from build123d import *

# Parameters (mm, degrees)
SKETCH1_W           = 94
SKETCH1_H           = 57
BOSS_EXTRUDE1_DEPTH = 1
BOSS_EXTRUDE3_DEPTH = 30
SKETCH5_W           = 0.7
SKETCH5_H           = 1
BOSS_EXTRUDE4_DEPTH = 92
SKETCH6_W           = 47
SKETCH6_H           = 10
CUT_EXTRUDE2_DEPTH  = 30
SKETCH7_W           = 10
SKETCH7_H           = 2
BOSS_EXTRUDE5_DEPTH = 2


with BuildPart() as part:
    # Sketch1 → Boss-Extrude1 (new body)
    with BuildSketch(Plane(origin=(0, 0, 0), x_dir=(1, 0, 0), z_dir=(0, 1, 0))):
        with Locations((-9.450515464, -3.911340206)):
            Rectangle(SKETCH1_W, SKETCH1_H)
    extrude(amount=BOSS_EXTRUDE1_DEPTH)

    # Sketch2 → Boss-Extrude3 (add)
    with BuildSketch(Plane(origin=(0, 1, 0), x_dir=(1, 0, 0), z_dir=(0, 1, 0))):
        Polygon((-56.450515464, 24.588659794), (37.549484536, 24.588659794), (37.549484536, -32.411340206), (-56.450515464, -32.411340206), (-56.450515464, -30.411340206), (-54.450515464, -30.411340206), (35.549484536, -30.411340206), (35.549484536, 22.588659794), (-54.450515464, 22.588659794), (-56.450515464, 22.588659794), align=None)
    extrude(amount=BOSS_EXTRUDE3_DEPTH)

    # Sketch5 → Boss-Extrude4 (add)
    with BuildSketch(Plane.ZY.offset(56.450515464)):
        with Locations((-22.238659794, 5.5)):
            Rectangle(SKETCH5_W, SKETCH5_H)
        with Locations((30.061340206, 5.5)):
            Rectangle(SKETCH5_W, SKETCH5_H)
    extrude(amount=-BOSS_EXTRUDE4_DEPTH)

    # Sketch6 → Cut-Extrude2 (cut)
    with BuildSketch(Plane(origin=(0, 0, -24.588659794), x_dir=(-1, 0, 0), z_dir=(0, 0, -1))):
        with Locations((-7.049484536, 19.5)):
            Rectangle(SKETCH6_W, SKETCH6_H)
    extrude(amount=-CUT_EXTRUDE2_DEPTH, mode=Mode.SUBTRACT)

    # Sketch7 → Boss-Extrude5 (add)
    with BuildSketch(Plane(origin=(0, 31, 0), x_dir=(1, 0, 0), z_dir=(0, 1, 0))):
        with Locations((-51.450515464, 23.588659794)):
            Rectangle(SKETCH7_W, SKETCH7_H)
        with Locations((-23.450515464, 23.588659794)):
            Rectangle(SKETCH7_W, SKETCH7_H)
        with Locations((4.549484536, 23.588659794)):
            Rectangle(SKETCH7_W, SKETCH7_H)
        with Locations((32.549484536, 23.588659794)):
            Rectangle(SKETCH7_W, SKETCH7_H)
        with Locations((-51.450515464, -31.411340206)):
            Rectangle(SKETCH7_W, SKETCH7_H)
        with Locations((-23.450515464, -31.411340206)):
            Rectangle(SKETCH7_W, SKETCH7_H)
        with Locations((4.549484536, -31.411340206)):
            Rectangle(SKETCH7_W, SKETCH7_H)
        with Locations((32.549484536, -31.411340206)):
            Rectangle(SKETCH7_W, SKETCH7_H)
    extrude(amount=BOSS_EXTRUDE5_DEPTH)


solid = part.part
Here's how the part is built. I have some questions about the finished solid (model axes, mm). A direction names the side the tool comes from. Give positions to 0.01 mm unless a question says otherwise; leave off trailing zeros. Loops run counter-clockwise (first coordinate to the right, second up) from the corner with the lowest first, then second, coordinate; pieces in that order, holes last. Notation, with made-up numbers: (84.5, 46) -> (108.5, 46) arc R25 ccw to (108.5, 81) -> close; hole circle Ø2 at (20, 35.5). An arc over 180 degrees is marked (long way). Answer as a JSON object with one key per item and string values. Group by question number.
Item 1: I need wall thicknesses on L1, parallel to Z at x = -4, y = 3.5; L2, parallel to Z at x = 14, y = 17.5; L3, parallel to Y at x = -33, z = 13. Which ranges of each line are inside material? Lowest first, please.
Item 2: Imagine slicing it at A-A on x = 10.5. Write out the boundary of the cut face in (y, z), then the cut area to 3 significant figures.
Item 3: On a 3-axis mill with a long thin cutter (end or side, diameter ignored), from which of +Z, -Z, +X, -X, +Y, -Y can I reach the whole of each face in a straight line? I mean faces 4 (the flat face through (37, 31, 4)), 5 (the flat face through (9.549, 32, -24)), 6 (the flat face through (-52, 33, 31)), 7 (the flat face through (7, 14.5, -24)), 8 (the flat face through (-11, 3, -22.589)). Say none if no direction works.
Item 4: Imagine slicing it at D-D on y = 7. Write out the boundary of the cut face in (x, z).
Item 5: Will these pins go through, and if not, where does the flat tip stop? pin 1 (2 mm diameter, centred on x = 15, z = -23.5, fed in from +Y); pin 2 (8 mm diameter, centred on y = 28, z = -12, fed in from -X).
Item 6: Imagine slicing it at C-C on z = -4.5. Write out the boundary of the cut face in (x, y).
Item 7: Imagine slicing it at B-B on y = 18.5. Write out the boundary of the cut face in (x, z).
Item 8: Thinking about a two-plate mould opening in Z: for faces 1 (the flat face through (37.549, 16, 4)), 2 (the flat face through (-10, 13, -22.589)), 3 (the flat face through (-9, 16, 32.411)), which applies, pulls with the +Z half, pulls with the -Z half, needs draft (parallel to the pull), parting line crosses it, or undercut?
Answer list:
{
 "1": {"L1": "z = -24.59 to -22.59, 30.41 to 32.41", "L2": "z = 30.41 to 32.41", "L3": "y = 0 to 1"},
 "2": {"outline": "(0, -24.59) -> (14.5, -24.59) -> (14.5, -22.59) -> (6, -22.59) -> (6, -21.89) -> (5, -21.89) -> (5, -22.59) -> (1, -22.59) -> (1, 30.41) -> (5, 30.41) -> (5, 29.71) -> (6, 29.71) -> (6, 30.41) -> (31, 30.41) -> (31, 32.41) -> (0, 32.41) -> close; (24.5, -24.59) -> (31, -24.59) -> (31, -22.59) -> (24.5, -22.59) -> close", "area": "158 mm2"},
 "3": {"face 4": "+X, -X, +Y", "face 5": "+Z, -Z, +Y", "face 6": "+Z, -Z, +X, -X, +Y", "face 7": "-Z", "face 8": "-X"},
 "4": {"outline": "(-56.45, -24.59) -> (37.55, -24.59) -> (37.55, 32.41) -> (-56.45, 32.41) -> (-56.45, 30.41) -> (35.55, 30.41) -> (35.55, -22.59) -> (-56.45, -22.59) -> close"},
 "5": {"pin 1": "stops at y = 31", "pin 2": "stops at x = 35.55"},
 "6": {"outline": "(-56.45, 0) -> (37.55, 0) -> (37.55, 31) -> (35.55, 31) -> (35.55, 1) -> (-56.45, 1) -> close"},
 "7": {"outline": "(-56.45, -24.59) -> (-16.45, -24.59) -> (-16.45, -22.59) -> (-56.45, -22.59) -> close; (-56.45, 30.41) -> (35.55, 30.41) -> (35.55, -22.59) -> (30.55, -22.59) -> (30.55, -24.59) -> (37.55, -24.59) -> (37.55, 32.41) -> (-56.45, 32.41) -> close"},
 "8": {"face 1": "needs draft", "face 2": "undercut", "face 3": "pulls with the +Z half"}
}
